Geometry: see drawing. Coordinates: mm, zero at the bounding-box minimum. Coordinates: 2 decimals unless noted, no trailing zeros. Loops run counter-clockwise (first coordinate to the right, second up) from the corner with the lowest first, then second, coordinate; pieces in that order, holes last. Notation, with made-up numbers: M -10,-2.75 L 13,-2.75 A14 ccw 13,9.25 Z; hole C -6.5,19 d6. An arc over 180 degrees is marked long. One line per question, with ' | ' between items. Start each with the question number.
1. Section query A-A, the plane x = 6. Output: boundary loops of the cut face in (y, z).
2. Pin query (flat end, axial travel): P1, Ø5.5, axis at x = 6, y = 6, coming from the +Z side; P2, Ø1.5, axis at y = 4.5, z = 5.5, coming from the +X side. Return the tip coordinate at first contact, or that it passes through.
3. Ray query, probe 1 along Y at (x, z) = (10.85, 10); probe 2 along X at (y, z) = (7.5, 3.25); probe 3 along Y at (x, z) = (3.75, 9.75). Return the intervals inside material, ascending.
4. Section query D-D, the plane z = 5. Output: boundary loops of the cut face in (x, y), and give its area (3 significant figures).
5. Mould query, pull axis Y, two halves, no side actions, for the marked faces 1, 2 and 3. Classes: pulls with the +Y half, pulls with the -Y half, needs draft (parallel to the pull), parting line crosses it, or undercut.
6. Section query B-B, the plane y = 6. Output: boundary loops of the cut face in (x, z).
7. Section query C-C, the plane y = 3.25. Output: boundary loops of the cut face in (x, z), and give its area (3 significant figures).
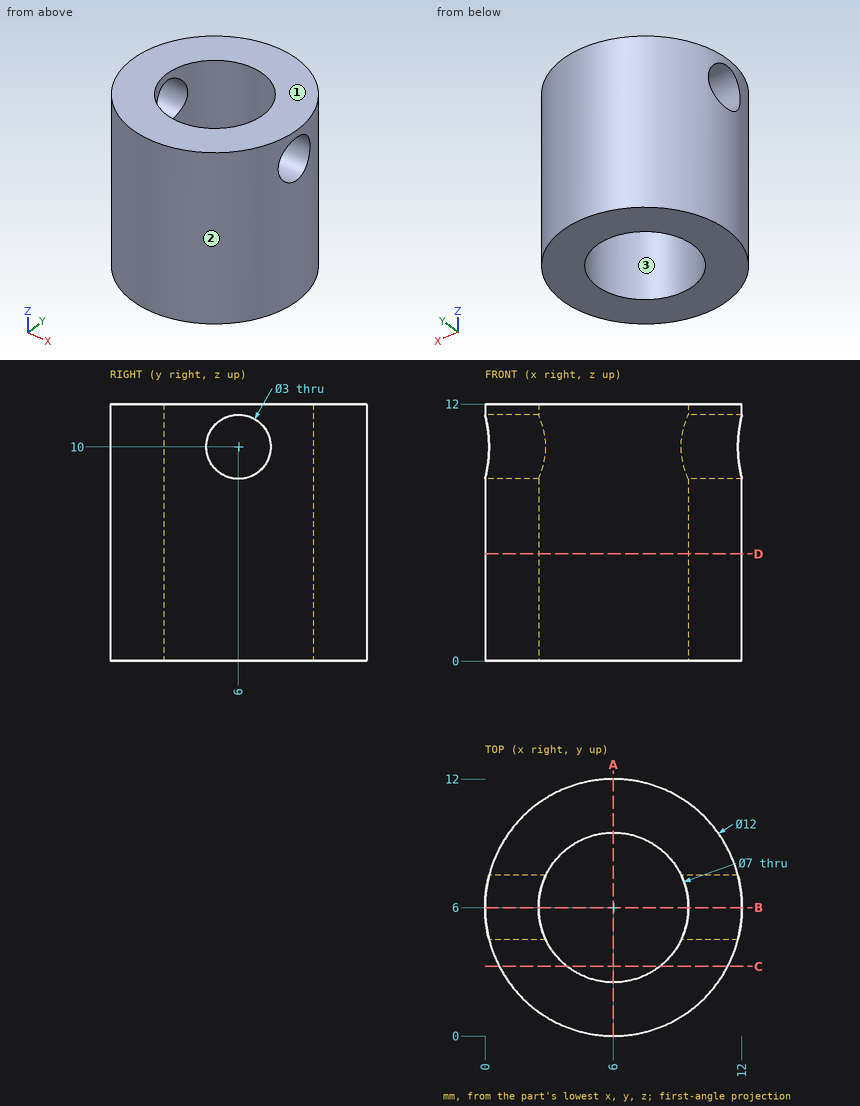
Taken from the geometry:
1) outline: M 0,0 L 2.5,0 L 2.5,12 L 0,12 Z; M 9.5,0 L 12,0 L 12,12 L 9.5,12 Z
2) P1: through | P2: x = 11.95
3) probe 1: 2.47 to 4.5, 7.5 to 9.53 | probe 2: 0.19 to 2.84, 9.16 to 11.81 | probe 3: 0.44 to 3.32, 8.68 to 11.56
4) outline: C 6,6 d12; hole C 6,6 d7 | area: 74.6 mm^2
5) face 1: needs draft | face 2: parting line crosses it | face 3: undercut
6) outline: M 0,0 L 2.5,0 L 2.5,8.5 L 0,8.5 Z; M 0,11.5 L 2.5,11.5 L 2.5,12 L 0,12 Z; M 9.5,0 L 12,0 L 12,8.5 L 9.5,8.5 Z; M 9.5,11.5 L 12,11.5 L 12,12 L 9.5,12 Z
7) outline: M 0.67,0 L 3.83,0 L 3.83,12 L 0.67,12 Z; M 8.17,0 L 11.33,0 L 11.33,12 L 8.17,12 Z | area: 76.0 mm^2
